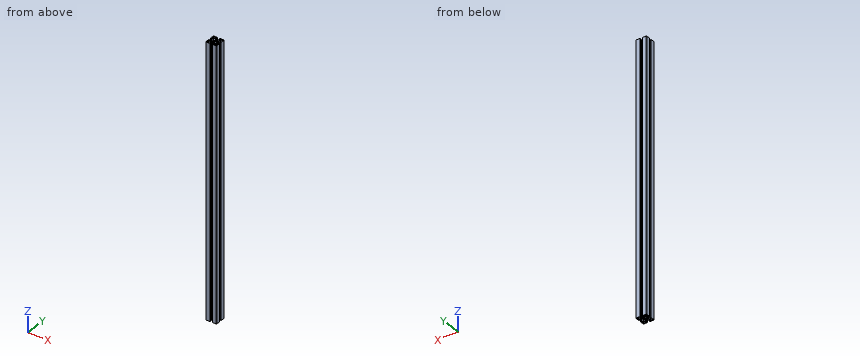
```python
from build123d import *

# Parameters (mm, degrees)
SKETCH1_R           = 3.4
SKETCH1_W           = 7.85
SKETCH1_H           = 7.85
BOSS_EXTRUDE1_DEPTH = 1000


with BuildPart() as part:
    # Sketch1 → Boss-Extrude1 (new body)
    with BuildSketch(Plane.XY):
        with BuildLine():
            Line((-7.15, 16), (-4.15, 16))
            Line((-4.15, 16), (-4.15, 20))
            Line((-4.15, 20), (-18.5, 20))
            ThreePointArc((-18.5, 20), (-19.560660172, 19.560660172), (-20, 18.5))
            Line((-20, 18.5), (-20, 4.15))
            Line((-20, 4.15), (-16, 4.15))
            Line((-16, 4.15), (-16, 7.15))
            Line((-16, 7.15), (-9, 7.15))
            Line((-9, 7.15), (-9, 4.15))
            Line((-9, 4.15), (-6, 4.15))
            Line((-6, 4.15), (-6, 0.519615242))
            Line((-6, 0.519615242), (-5.7, 0))
            Line((-5.7, 0), (-6, -0.519615242))
            Line((-6, -0.519615242), (-6, -4.15))
            Line((-6, -4.15), (-9, -4.15))
            Line((-9, -4.15), (-9, -7.15))
            Line((-9, -7.15), (-16, -7.15))
            Line((-16, -7.15), (-16, -4.15))
            Line((-16, -4.15), (-20, -4.15))
            Line((-20, -4.15), (-20, -18.5))
            ThreePointArc((-20, -18.5), (-19.560660172, -19.560660172), (-18.5, -20))
            Line((-18.5, -20), (-4.15, -20))
            Line((-4.15, -20), (-4.15, -16))
            Line((-4.15, -16), (-7.15, -16))
            Line((-7.15, -16), (-7.15, -9))
            Line((-7.15, -9), (-4.15, -9))
            Line((-4.15, -9), (-4.15, -6))
            Line((-4.15, -6), (-0.519615242, -6))
            Line((-0.519615242, -6), (0, -5.7))
            Line((0, -5.7), (0.519615242, -6))
            Line((0.519615242, -6), (4.15, -6))
            Line((4.15, -6), (4.15, -9))
            Line((4.15, -9), (7.15, -9))
            Line((7.15, -9), (7.15, -16))
            Line((7.15, -16), (4.15, -16))
            Line((4.15, -16), (4.15, -20))
            Line((4.15, -20), (18.5, -20))
            ThreePointArc((18.5, -20), (19.560660172, -19.560660172), (20, -18.5))
            Line((20, -18.5), (20, -4.15))
            Line((20, -4.15), (16, -4.15))
            Line((16, -4.15), (16, -7.15))
            Line((16, -7.15), (9, -7.15))
            Line((9, -7.15), (9, -4.15))
            Line((9, -4.15), (6, -4.15))
            Line((6, -4.15), (6, -0.519615242))
            Line((6, -0.519615242), (5.7, 0))
            Line((5.7, 0), (6, 0.519615242))
            Line((6, 0.519615242), (6, 4.15))
            Line((6, 4.15), (9, 4.15))
            Line((9, 4.15), (9, 7.15))
            Line((9, 7.15), (16, 7.15))
            Line((16, 7.15), (16, 4.15))
            Line((16, 4.15), (20, 4.15))
            Line((20, 4.15), (20, 18.5))
            ThreePointArc((20, 18.5), (19.560660172, 19.560660172), (18.5, 20))
            Line((18.5, 20), (4.15, 20))
            Line((4.15, 20), (4.15, 16))
            Line((4.15, 16), (7.15, 16))
            Line((7.15, 16), (7.15, 9))
            Line((7.15, 9), (4.15, 9))
            Line((4.15, 9), (4.15, 6))
            Line((4.15, 6), (0.519615242, 6))
            Line((0.519615242, 6), (0, 5.7))
            Line((0, 5.7), (-0.519615242, 6))
            Line((-0.519615242, 6), (-4.15, 6))
            Line((-4.15, 6), (-4.15, 9))
            Line((-4.15, 9), (-7.15, 9))
            Line((-7.15, 9), (-7.15, 16))
        make_face()
        with Locations(Location((0, 0, 0), (0, 0, 180))):
            Circle(SKETCH1_R, mode=Mode.SUBTRACT)
        with Locations((-13.575, 13.575)):
            Rectangle(SKETCH1_W, SKETCH1_H, mode=Mode.SUBTRACT)
        with Locations((13.575, 13.575)):
            Rectangle(SKETCH1_W, SKETCH1_H, mode=Mode.SUBTRACT)
        with Locations((-13.575, -13.575)):
            Rectangle(SKETCH1_W, SKETCH1_H, mode=Mode.SUBTRACT)
        with Locations((13.575, -13.575)):
            Rectangle(SKETCH1_W, SKETCH1_H, mode=Mode.SUBTRACT)
    extrude(amount=-BOSS_EXTRUDE1_DEPTH)


solid = part.part
```
Work out the finished part from the listing and answer in its coordinate system (mm). Give positions to 0.01 mm unless a question says otherwise; leave off trailing zeros. Write item = value, one per line. Start each with the question number.
(1) Find section A-A on z = -519. Give the number of separate pieces and of enclosed holes in the cut face, and give its area (3 significant figures).
(2) Given pin 1 Ø5 at (x, y) = (7.5, 10) entering from +Z; pin 2 Ø1.8 at (y, z) = (3, -619) entering from -X; pin 3 Ø1.5 at (x, y) = (-5.5, -11) entering from -Z; pin 4 Ø1.8 at (x, z) = (3, -270) entering from -Y, each flat-ended and moving along its own axis, determine where each tip first touches the part or whether it passes through.
(3) Find the intervals of material crossed by probe 1 along X at (y, z) = (-15, -248); probe 2 along Y at (x, z) = (17, -697), in increasing order. Write a range as from..to.
From the geometry:
q1.separate_pieces = 1
q1.enclosed_holes = 5
q1.area = 682 mm^2
q2.pin_1 = 0
q2.pin_2 = -6
q2.pin_3 = through
q2.pin_4 = -6
q3.probe_1 = -20..-17.5, -9.65..-7.15, 7.15..9.65, 17.5..20
q3.probe_2 = -20..-17.5, -9.65..-4.15, 4.15..9.65, 17.5..20
